from build123d import *

# Parameters (mm, degrees)
CROQUIS1_W              = 101.6
CROQUIS1_H              = 50.8
SALIENTE_EXTRUIR1_DEPTH = 6.31
CROQUIS2_R              = 4.7625
CORTAR_EXTRUIR1_DEPTH   = 6.31
MATRIZL1_COUNT          = 2
MATRIZL1_PITCH          = 50.8


with BuildPart() as part:
    # Croquis1 → Saliente-Extruir1 (new body)
    with BuildSketch(Plane(origin=(0, 0, 0), x_dir=(1, 0, 0), z_dir=(0, 1, 0))):
        Rectangle(CROQUIS1_W, CROQUIS1_H)
    extrude(amount=SALIENTE_EXTRUIR1_DEPTH)

    # Croquis2 → Cortar-Extruir1 (cut)
    with BuildSketch(Plane(origin=(0, 6.31, 0), x_dir=(1, 0, 0), z_dir=(0, 1, 0))):
        with Locations(Location((-38.1, -12.7, 0), (0, 0, 270))):
            Circle(CROQUIS2_R)
        with Locations(Location((-12.7, 12.7, 0), (0, 0, 270))):
            Circle(CROQUIS2_R)
    cortar_extruir1 = extrude(amount=-CORTAR_EXTRUIR1_DEPTH, mode=Mode.SUBTRACT)

    # MatrizL1: Cortar-Extruir1 ×2
    with Locations(*[(i * MATRIZL1_PITCH, 0, 0) for i in range(1, MATRIZL1_COUNT)]):
        add(cortar_extruir1, mode=Mode.SUBTRACT)


solid = part.part
Can you work these out from the model? Positions are in its coordinate system, mm. Coordinates: 2 decimals unless noted, no trailing zeros. Order: outer loops, then holes, each group sorted by start corner. A loop starts at its lowest first (then second) coordinate and runs counter-clockwise, first axis right, second up. Notation, with made-up numbers: M -39,30 L -30,30 A29 ccw -30,54 Z; hole C 4,-7 d10. An arc over 180 degrees is marked long. Answer as CSV lines item,"result".
(1) Please list where these lines run through material, in increasing order: L1, parallel to X at y = 4.75, z = 12.7; L2, parallel to X at y = 4.5, z = -16; L3, parallel to Z at x = 15, y = 5.5.
Geometry check:
L1,"-50.8 to -42.86, -33.34 to 7.94, 17.46 to 50.8"
L2,"-50.8 to -16.13, -9.27 to 34.67, 41.53 to 50.8"
L3,"-25.4 to 8.53, 16.87 to 25.4"
(2) Suppose I cut it at C-C on x = -38.1. Please give me the cut outline in (y, z).
Geometry check:
outline,"M 0,-25.4 L 6.31,-25.4 L 6.31,7.94 L 0,7.94 Z; M 0,17.46 L 6.31,17.46 L 6.31,25.4 L 0,25.4 Z"
(3) Suppose I cut it at D-D on x = -10. Please give me the cut outline in (y, z), plus the area to 3 significant figures.
Geometry check:
outline,"M 0,-25.4 L 6.31,-25.4 L 6.31,-16.62 L 0,-16.62 Z; M 0,-8.78 L 6.31,-8.78 L 6.31,25.4 L 0,25.4 Z"
area,"271 mm^2"
(4) Suppose I cut it at A-A on z = -12.7. Please give me the cut outline in (x, y).
Geometry check:
outline,"M -50.8,0 L -17.46,0 L -17.46,6.31 L -50.8,6.31 Z; M -7.94,0 L 33.34,0 L 33.34,6.31 L -7.94,6.31 Z; M 42.86,0 L 50.8,0 L 50.8,6.31 L 42.86,6.31 Z"
(5) Suppose I cut it at B-B on y = 2. Please give me the cut outline in (x, z) (1 decimal), plus the area to 3 significant figures.
Geometry check:
outline,"M -50.8,-25.4 L 50.8,-25.4 L 50.8,25.4 L -50.8,25.4 Z; hole C -38.1,12.7 d9.5; hole C -12.7,-12.7 d9.5; hole C 12.7,12.7 d9.5; hole C 38.1,-12.7 d9.5"
area,"4,880 mm^2"
(6) I'm going to push a flat-ended pin straight in: pin 1 (7.5 mm diameter, centred on x = 38.1, z = -12.7, fed in from +Y). Where does the tip first touch, or does it pass through?
Geometry check:
pin 1,"through"
(7) If we mould it in two halves opening along X, with no side actions, what happens to faces 1 (the flat face through (50.8, 3, 0)), 2 (the flat face through (-1, 0, 0)), 3 (the flat face through (-50.8, 3, 0)), 4 (the cylindrical face through (-11.269, 3.199, -8.157))? For each: released by +X, released by -X, zero draft, split by the parting line, or undercut.
Geometry check:
face 1,"released by +X"
face 2,"zero draft"
face 3,"released by -X"
face 4,"undercut"
